Build history of the part. All positions in model axes, mm. A direction names the side the tool comes from. Give positions to 0.01 mm unless a question says otherwise; leave off trailing zeros. Loops run counter-clockwise (first coordinate to the right, second up) from the corner with the lowest first, then second, coordinate; pieces in that order, holes last.
1) Wall check: line 1 (Z direction, x = -6.5, y = -3.25); line 2 (Z direction, x = -3.5, y = -6). Give the ranges that are in metal, low to high.
2) Band-saw the part on A-A on x = 0.75. List the corners of the cut face in (y, z).
3) Flat gauge pins, fed straight in: P1, Ø2, axis at y = -3.18, z = 96.83, coming from the +X side; P2, Ø1.9, axis at x = 0, y = -3.5, coming from the +Z side; P3, Ø3, axis at x = 2, z = 11.5, coming from the +Y side. Where does each tip first touch, or does it go through?
4) Two-plate mould, pull along X, no slides. Class faces 3 (the flat face through (2.515, -5, 97)), 4 (the flat face through (-7.645, -3, 36)), 5 (the cylindrical face through (3.8, -3.34, 98.09)): +X half, -X half, draft (parallel to the pull), parting line (faces both ways), or undercut.
5) 3-axis set-ups, long thin cutter, end or side, ignore diameter. For faces 1 (the flat face through (-5.105, -5, 97)), 2 (the flat face through (-1, 0, 37)): which of +Z, -Z, +X, -X, +Y, -Y reach the whole face in a straight line?
```python
from build123d import *

# Parameters (mm, degrees)
F0_W     = 12.7
F0_H     = 127
F1_DEPTH = 6.35
F2_W     = 7.62
F2_H     = 6.35
F3_DEPTH = 6.351
F4_R     = 1.27
F5_DEPTH = 12.7


with BuildPart() as f1:
    # F0 (on Front) → F1 (new body)
    with BuildSketch(Plane.XZ):
        with Locations((-1.295127, 36.507539)):
            Rectangle(F0_W, F0_H)
    extrude(amount=F1_DEPTH)

    # F2 (on Front) → F3 (cut, through all)
    with BuildSketch(Plane.XZ):
        with Locations((-1.295127, 96.832539)):
            Rectangle(F2_W, F2_H)
    extrude(amount=F3_DEPTH, mode=Mode.SUBTRACT)

    # F4 (on face) → F5 (cut, symmetric)
    with BuildSketch(Plane.YZ.offset(-5.105127)):
        with Locations((-3.175, 96.832539)):
            Circle(F4_R)
    extrude(amount=F5_DEPTH, both=True, mode=Mode.SUBTRACT)


solid = f1.part
```
Findings below:
1. line 1: z = -26.99 to 95.56, 98.1 to 100.01
1. line 2: z = -26.99 to 93.66
2. outline: (-6.35, -26.99) - (0, -26.99) - (0, 93.66) - (-6.35, 93.66) - close
3. P1: passes through
3. P2: stops at z = 93.66
3. P3: stops at y = 0
4. face 3: undercut
4. face 4: -X half
4. face 5: draft
5. face 1: +Z, +Y, -Y
5. face 2: +Z, -Z, +X, -X, +Y
